Work out the finished part from the listing and answer in its coordinate system (mm). Face numbers are marked on the shaded views. A direction names the side the tool comes from. Give positions to 0.01 mm unless a question says otherwise; leave off trailing zeros. Write each loop counter-clockwise with the first axis right and the second up, starting at its lowest first coordinate (ties: lowest second). Pieces come first, ordered by that corner, then holes. Notation, with made-up numbers: (-22.5, 20) - (-6.5, 20) arc R17 ccw to (-6.5, 51) - close; hole circle Ø2 at (28, -4.5). An arc over 180 degrees is marked (long way). Write item = value, one per line.
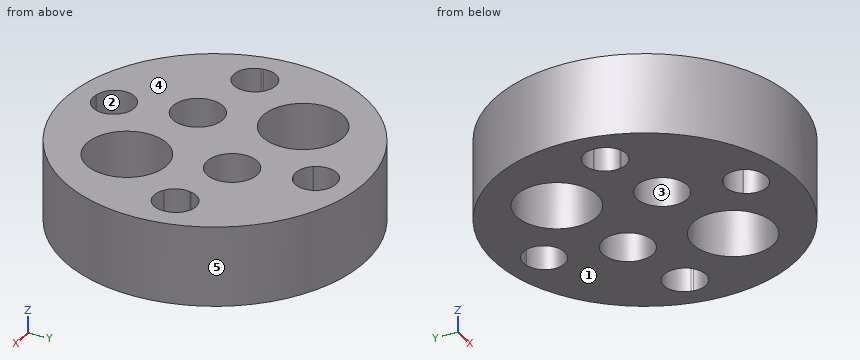
Autodesk Inventor part; units mm, degrees
ref_plane "YZ Plane" through (0, 0, 0) normal (1, 0, 0) x (0, 1, 0)
ref_plane "XZ Plane" through (0, 0, 0) normal (0, 1, 0) x (-1, 0, 0)
ref_plane "XY Plane" through (0, 0, 0) normal (0, 0, 1) x (1, 0, 0)
sketch "スケッチ1" plane through (0, 0, 0) normal (0, 0, 1) x (1, 0, 0)
  circle A0 centre (-12.0208, 12.0208) radius 9.5
  arc A1 (-18.7383, 18.7383) -> (-18.7383, -18.7383) centre (0, 0) ccw
  circle A2 centre (-14.8669, 14.8669) radius 2
  circle A3 centre (-10.253, 13.7886) radius 1.25
  circle A4 centre (-13.7886, 10.253) radius 1.25
  circle A5 centre (-9.1747, 9.1747) radius 2
  circle A6 centre (-12.0208, -12.0208) radius 9.5
  arc A7 (-8.2499, -13.092) -> (-13.092, -8.2499) centre (-9.1747, -9.1747) ccw
  circle A8 centre (-9.1747, -9.1747) radius 2
  circle A9 centre (-13.7886, -10.253) radius 1.25
  arc A10 (-13.9423, -9.0125) -> (-13.092, -8.2499) centre (-14.0653, -8.0201) ccw
  arc A11 (-15.7917, -10.9496) -> (-15.0291, -10.0993) centre (-16.0215, -9.9764) ccw
  arc A12 (-15.7917, -10.9496) -> (-10.9496, -15.7917) centre (-14.8669, -14.8669) ccw
  circle A13 centre (-14.8669, -14.8669) radius 2
  circle A14 centre (-10.253, -13.7886) radius 1.25
  arc A15 (-10.0993, -15.0291) -> (-10.9496, -15.7917) centre (-9.9764, -16.0215) ccw
  arc A16 (-10.0993, -15.0291) -> (-9.0125, -13.9423) centre (-10.253, -13.7886) ccw
  arc A17 (-8.2499, -13.092) -> (-9.0125, -13.9423) centre (-8.0201, -14.0653) ccw
  arc A18 (-7.6297, -14.4272) -> (-14.4272, -7.6297) centre (-9.1747, -9.1747) ccw
  arc A19 (-9.6145, -16.412) -> (-7.6297, -14.4272) centre (-10.253, -13.7886) ccw
  arc A20 (-16.412, -9.6145) -> (-9.6145, -16.412) centre (-14.8669, -14.8669) ccw
  arc A21 (-14.4272, -7.6297) -> (-16.412, -9.6145) centre (-13.7886, -10.253) ccw
  arc A22 (-11.6204, 16.1746) -> (-16.1746, 11.6204) centre (-14.8669, 14.8669) ccw
  arc A23 (-7.8671, 12.4213) -> (-11.6204, 16.1746) centre (-10.253, 13.7886) ccw
  arc A24 (-16.1746, 11.6204) -> (-12.4213, 7.8671) centre (-13.7886, 10.253) ccw
  arc A25 (-12.4213, 7.8671) -> (-7.8671, 12.4213) centre (-9.1747, 9.1747) ccw
  circle A26 centre (-12.0208, -12.0208) radius 8
  line L0 (-25.4165, 7.5) -> (-25.4165, -7.5)
  line L1 (-23.9165, 7.2801) -> (-23.9165, -7.2801)
  arc A27 (-21.491, 12.7724) -> (-23.9165, 7.2801) centre (0, 0) ccw
  arc A28 (-23.9165, -7.2801) -> (-21.491, -12.7724) centre (0, 0) ccw
  line L2 (-2.5208, 12.0208) -> (-2.5208, -12.0208)
  line L3 (-4.0208, 6.8973) -> (-4.0208, -6.8973)
  circle A29 centre (-12.0208, 12.0208) radius 7.5
  line L4 (-13.7886, -10.253) -> (-4.0461, -19.9955) construction
  line L5 (-13.7886, 10.253) -> (-4.0869, 19.9547) construction
  line L6 (-12.7708, 2.5505) -> (-12.7708, -2.5505)
  line L7 (-11.2708, 2.5505) -> (-11.2708, -2.5505)
  arc A30 (-10.8714, 16.4682) -> (-10.9282, 18.4283) centre (-11.0963, 17.4426) ccw
  arc A31 (-5.6133, 13.1135) -> (-7.5735, 13.1702) centre (-6.5991, 12.9454) ccw
  arc A32 (-13.1702, 7.5735) -> (-13.1135, 5.6133) centre (-12.9454, 6.5991) ccw
  arc A33 (-18.4283, 10.9282) -> (-16.4682, 10.8714) centre (-17.4426, 11.0963) ccw
  arc A34 (-10.9282, 18.4283) -> (-13.9213, 18.2368) centre (-12.0208, 12.0208) ccw
  arc A35 (-18.2368, 13.9213) -> (-18.4283, 10.9282) centre (-12.0208, 12.0208) ccw
  arc A36 (-13.1135, 5.6133) -> (-10.1203, 5.8049) centre (-12.0208, 12.0208) ccw
  arc A37 (-5.8049, 10.1203) -> (-5.6133, 13.1135) centre (-12.0208, 12.0208) ccw
  point P0 (0, 0)
  point P1 (0, 0)
  point P2 (-5.3033, -18.7383)
  point P3 (-5.3033, 18.7383)
  dimension "d0" = 1.45
  dimension "d1" = 1.45
  dimension "d2" = 1.5
  dimension "d3" = 1.5
  dimension "d4" = 1.5
  dimension "d5" = 1.5
  dimension "d6" = 1.5
  dimension "d7" = 15
  dimension "d8" = 1.5
  dimension "d9" = 1.5
  dimension "d10" = 1.5
  dimension "d11" = 1.5
  dimension "d12" = 15
  dimension "d13" = 1.5
  dimension "d14" = 0.75
  dimension "d16" = 2
  dimension "d17" = 2
  dimension "d18" = 2
  dimension "d19" = 2
  dimension "d23" = 4
  dimension "d24" = 4
  dimension "d25" = 1
  dimension "d26" = 1
  dimension "d27" = 1
  dimension "d28" = 1
extrude "押し出し1" add sketch "スケッチ1" along normal blind 4 contours A23 A25 A29 A24 A22 | A22 A29 A25 A37 A31 A23 A30 A34 | A22 A35 A33 A24 A32 A36 A25 A29
fillet "フィレット1" radius 1 8 edges at (-10.1203, 5.8049, 2) (-12.4213, 7.8671, 2) (-16.1746, 11.6204, 2) (-18.2368, 13.9213, 2) (-7.8671, 12.4213, 2) (-5.8049, 10.1203, 2) (-13.9213, 18.2368, 2) (-11.6204, 16.1746, 2)
properties part number "新型３脚カム" material "アルミニウム 7075"
1. Straight lines are drawn through the part: line 1 (Y direction, x = -13.25, z = 1.9); line 2 (X direction, y = 11.25, z = 2.25); line 3 (Y direction, x = -9.5, z = 3.15). For each, find the intervals that lie inside material, in ascending order.
Solution:
line_1 = 4.62 to 5.65, 7.55 to 9.12, 11.38 to 13.69, 16.04 to 19.42
line_2 = -19.48 to -18.46, -16.43 to -14.54, -13.03 to -4.56
line_3 = 4.96 to 7.2, 11.15 to 12.79, 14.79 to 19.08
2. Given pin 1 (2 mm diameter, centred on x = -8.5, z = 1, fed in from -Y); pin 2 (2 mm diameter, centred on x = -18, z = 2.5, fed in from -Y); pin 3 (1 mm diameter, centred on x = -8, z = 1.5, fed in from -Y), each flat-ended and moving along its own axis, determine where each tip first touches the part or whether it passes through.
Solution:
pin_1 = 4.96
pin_2 = 6.41
pin_3 = 5.4
3. Find section A-A, the plane x = -14.5. Give the vertices of the cut face in (y, z), then the cut area to 3 significant figures.
Solution:
outline = (4.94, 0) - (9.23, 0) - (9.23, 4) - (4.94, 4) - close; (11.28, 0) - (12.9, 0) - (12.9, 4) - (11.28, 4) - close; (16.83, 0) - (19.1, 0) - (19.1, 4) - (16.83, 4) - close
area = 32.7 mm^2
4. Find section B-B, the plane y = 14.5. Give the vertices of the cut face in (x, z), then the cut area to 3 significant figures.
Solution:
outline = (-19.1, 0) - (-16.83, 0) - (-16.83, 4) - (-19.1, 4) - close; (-12.9, 0) - (-11.28, 0) - (-11.28, 4) - (-12.9, 4) - close; (-9.23, 0) - (-4.94, 0) - (-4.94, 4) - (-9.23, 4) - close
area = 32.7 mm^2
5. A tool of negligible diameter and unlimited length cuts with its end or side. For the marked faces 1 and 2, from which of +Z, -Z, +X, -X, +Y, -Y can it reach the whole face along a straight path? Write none if from no direction.
Solution:
face_1 = -Z, +X, -X, +Y, -Y
face_2 = +Z, -Z
6. For a pull along Y with two mould halves and no side action, classify the marked faces 3, 4 and 5 as pulls with the +Y half, pulls with the -Y half, needs draft (parallel to the pull), parting line crosses it, or undercut.
Solution:
face_3 = undercut
face_4 = needs draft
face_5 = parting line crosses it
7. Find section C-C, the plane z = 3.15. Give the number of separate pieces and of enclosed holes in the cut face, then the cut area to 3 significant figures.
Solution:
separate_pieces = 1
enclosed_holes = 8
area = 128 mm^2
